```python
from build123d import *

# Parameters (mm, degrees)
SKETCH1_W           = 635
SKETCH1_H           = 190.5
BOSS_EXTRUDE1_DEPTH = 12.7
SKETCH2_R           = 9.525
CUT_EXTRUDE1_DEPTH  = 332.72293032


with BuildPart() as part:
    # Sketch1 → Boss-Extrude1 (new body)
    with BuildSketch(Plane(origin=(0, 0, 0), x_dir=(1, 0, 0), z_dir=(0, 1, 0))):
        Rectangle(SKETCH1_W, SKETCH1_H)
    extrude(amount=-BOSS_EXTRUDE1_DEPTH)

    # Sketch2 → Cut-Extrude1 (cut, through all)
    with BuildSketch(Plane(origin=(0, 0, 0), x_dir=(1, 0, 0), z_dir=(0, 1, 0))):
        with Locations(Location((0, 73.025, 0), (0, 0, 270))):
            Circle(SKETCH2_R)
    extrude(amount=-CUT_EXTRUDE1_DEPTH, mode=Mode.SUBTRACT)


solid = part.part
```
Part model, mm, in its own coordinate system. Round coordinates to 2 decimals unless told otherwise and drop trailing zeros. Write each loop counter-clockwise with the first axis right and the second up, starting at its lowest first coordinate (ties: lowest second). Pieces come first, ordered by that corner, then holes. Notation, with made-up numbers: (-3.75, -7.5) -> (36.25, -7.5) arc R23 cw to (36.25, 28.5) -> close; hole circle Ø1 at (73, 70.5). An arc over 180 degrees is marked (long way). Return JSON: item names as keys, results as strings. Group by question number.
Q1. Saw through at A-A on x = 0. Write the cut outline in (y, z), plus the area to 3 significant figures.
Q2. Mould opens along Z. For faces 1 (the cylindrical face through (2.86, -6.26, -63.94)), 2 (the flat face through (-4, -6, -95.25)), 3 (the flat face through (-4, -6, 95.25)), 4 (the flat face through (-317.5, -6, 1)) say: pulls with the +Z half, pulls with the -Z half, needs draft (parallel to the pull), parting line crosses it, or undercut.
Q3. Probe L1, parallel to X at y = -11.75, z = -79. List the from-to ranges inside material, lowest first. Write a range as [from, to].
Answer:
{
 "1": {"outline": "(-12.7, -95.25) -> (0, -95.25) -> (0, -82.55) -> (-12.7, -82.55) -> close; (-12.7, -63.5) -> (0, -63.5) -> (0, 95.25) -> (-12.7, 95.25) -> close", "area": "2,180 mm2"},
 "2": {"face 1": "undercut", "face 2": "pulls with the -Z half", "face 3": "pulls with the +Z half", "face 4": "needs draft"},
 "3": {"L1": "[-317.5, -7.42], [7.42, 317.5]"}
}
